Design review of the part built by this model. Coordinates are the model's own, in mm. A direction names the side the tool comes from. Round coordinates to 2 decimals unless told otherwise and drop trailing zeros. Order: outer loops, then holes, each group sorted by start corner. A loop starts at its lowest first (then second) coordinate and runs counter-clockwise, first axis right, second up. Notation, with made-up numbers: M -23.75,89.5 L 18.25,89.5 A8 cw 18.25,102.5 Z; hole C -9,-38.75 d7. An arc over 180 degrees is marked long. Use a Markdown table: item, result. Add a question column.
(1) Take a section at B-B (y = 0). Write out the cut boundary in (x, z).
(2) The part is to be moulded in two halves that separate along Z. For faces 4 (the face through (2.521, -48.656, 1.084)), 5 (the face through (-4, -36, 0)), 6 (the face through (0.06, -15.57, 7.88)), say which applies: released by +Z, released by -Z, zero draft, split by the parting line, or undercut.
(3) Take a section at C-C (x = -2). Write out the cut boundary in (y, z).
(4) Take a section at A-A (z = 0). Write out the cut boundary in (x, y).
(5) Take a section at D-D (y = -40). Write out the cut boundary in (x, z).
(6) To check wall thickness, follow probe 1 along Y at (x, z) = (1.8, 0); probe 2 along X at (y, z) = (-38, -7); probe 3 along Y at (x, z) = (0, -12.5). State the ranges of each line that lie inside material, in increasing order. Write a range as from..to.
(7) Machinability: for faces 1 (the face through (1, -42.6, 1.2)), 2 (the face through (0, -22, 7)), 3 (the face through (0.06, -15.57, -7.88)), which of the approach directions +Z, -Z, +X, -X, +Y, -Y give a long, thin tool a straight path to every point of the face, cutting with its end or side? Answer none if there is none.
(8) For pin 1 (2.5 mm diameter, centred on y = -43.77, z = 0, fed in from +X); pin 2 (2.5 mm diameter, centred on x = -0.5, y = -73.5, fed in from -Z); pin 3 (3.5 mm diameter, centred on x = 0, y = -22, fed in from +Z); pin 4 (8 mm diameter, centred on y = -43.77, z = 0, fed in from +X), all flat-tipped, find the tip position at first contact; note any pin that passes through.
```python
from build123d import *

# Parameters (mm, degrees)
BOSS_EXTRUDE1_DEPTH      = 4
BOSS_EXTRUDE1_DEPTH_BACK = 4
FILLET1_R                = 10
SKETCH2_R                = 5
CUT_EXTRUDE1_DEPTH       = 3
SKETCH3_R                = 1.5
CUT_EXTRUDE2_DEPTH       = 5
SKETCH4_R                = 18.5
CUT_EXTRUDE3_DEPTH       = 8
SKETCH5_R                = 21.5
SKETCH5_R_2              = 18.5
BOSS_EXTRUDE2_DEPTH      = 7


with BuildPart() as part:
    # Sketch1 → Boss-Extrude1 (new, two sides: drawn at the far end of the back side and taken through both)
    with BuildSketch(Plane(origin=(0, 0, 0), x_dir=(0, 0, -1), z_dir=(1, 0, 0)).offset(-BOSS_EXTRUDE1_DEPTH_BACK)):
        with BuildLine():
            Line((-7, -14.38749457), (-7, -29.38749457))
            ThreePointArc((-7, -29.38749457), (-16, -43.77498914), (-7, -58.16248371))
            Line((-7, -58.16248371), (-7, -88.16248371))
            ThreePointArc((-7, -88.16248371), (0, -129.99103506), (7, -88.16248371))
            Line((7, -88.16248371), (7, -58.16248371))
            ThreePointArc((7, -58.16248371), (16, -43.77498914), (7, -29.38749457))
            Line((7, -29.38749457), (7, -14.38749457))
            ThreePointArc((7, -14.38749457), (0, 16), (-7, -14.38749457))
        make_face()
    extrude(amount=BOSS_EXTRUDE1_DEPTH + BOSS_EXTRUDE1_DEPTH_BACK)

    # Fillet1
    fillet1_edges = [part.edges().sort_by_distance(p)[0] for p in [
        (0, -29.38749457, 7),
        (0, -14.38749457, 7),
        (0, -14.38749457, -7),
        (0, -29.38749457, -7),
        (0, -58.16248371, -7),
        (0, -88.16248371, -7),
        (0, -88.16248371, 7),
        (0, -58.16248371, 7),
    ]]
    fillet(fillet1_edges, radius=FILLET1_R)

    # Sketch2 → Cut-Extrude1 (cut)
    with BuildSketch(Plane(origin=(4, 0, 0), x_dir=(0, 0, -1), z_dir=(1, 0, 0))):
        Circle(SKETCH2_R)
        with Locations((0, -43.77498914)):
            Circle(SKETCH2_R)
    extrude(amount=-CUT_EXTRUDE1_DEPTH, mode=Mode.SUBTRACT)

    # Sketch3 → Cut-Extrude2 (cut)
    with BuildSketch(Plane(origin=(1, 0, 0), x_dir=(0, 0, -1), z_dir=(1, 0, 0))):
        Circle(SKETCH3_R)
        with Locations((0, -43.77498914)):
            Circle(SKETCH3_R)
    extrude(amount=-CUT_EXTRUDE2_DEPTH, mode=Mode.SUBTRACT)

    # Sketch4 → Cut-Extrude3 (cut)
    with BuildSketch(Plane(origin=(4, 0, 0), x_dir=(0, 0, -1), z_dir=(1, 0, 0))):
        with Locations((0, -108.49103506)):
            Circle(SKETCH4_R)
    extrude(amount=-CUT_EXTRUDE3_DEPTH, mode=Mode.SUBTRACT)

    # Sketch5 → Boss-Extrude2 (add)
    with BuildSketch(Plane.ZY.offset(4)):
        with Locations(Location((0, -108.49103506, 0), (0, 0, 122.662030563))):
            Circle(SKETCH5_R)
        with Locations(Location((0, -108.49103506, 0), (0, 0, 180))):
            Circle(SKETCH5_R_2, mode=Mode.SUBTRACT)
    extrude(amount=BOSS_EXTRUDE2_DEPTH)


solid = part.part
```
Verdict:
| question | item | result |
|---|---|---|
| 1 | outline | M -4,-16 L 4,-16 L 4,-5 L 1,-5 L 1,-1.5 L -4,-1.5 Z; M -4,1.5 L 1,1.5 L 1,5 L 4,5 L 4,16 L -4,16 Z |
| 2 | face 4 | undercut |
| 2 | face 5 | zero draft |
| 2 | face 6 | released by +Z |
| 3 | outline | M -90.39,-11.6 A10 cw -81.97,-7 L -63.45,-7 A10 cw -55.88,-10.46 A16 ccw -31.67,-10.46 A10 cw -24.1,-7 L -19.67,-7 A10 cw -12.11,-10.46 A16 ccw long -12.11,10.46 A10 cw -19.67,7 L -24.1,7 A10 cw -31.67,10.46 A16 ccw -55.88,10.46 A10 cw -63.45,7 L -81.97,7 A10 cw -90.39,11.6 A21.5 ccw long Z; hole C -108.49,0 d37; hole C -43.77,0 d3; hole C 0,0 d3 |
| 4 | outline | M -11,-129.99 L 4,-129.99 L 4,-126.99 L -11,-126.99 Z; M -11,-89.99 L 4,-89.99 L 4,-48.77 L 1,-48.77 L 1,-45.27 L -4,-45.27 L -4,-86.99 L -11,-86.99 Z; M -4,-42.27 L 1,-42.27 L 1,-38.77 L 4,-38.77 L 4,-5 L 1,-5 L 1,-1.5 L -4,-1.5 Z; M -4,1.5 L 1,1.5 L 1,5 L 4,5 L 4,16 L -4,16 Z |
| 5 | outline | M -4,-15.55 L 4,-15.55 L 4,-3.28 L 1,-3.28 L 1,3.28 L 4,3.28 L 4,15.55 L -4,15.55 Z |
| 6 | probe 1 | y = -129.99..-126.99, -89.99..-48.77, -38.77..-5, 5..16 |
| 6 | probe 2 | x = -4..4 |
| 6 | probe 3 | y = -125.98..-122.13, -94.85..-91, -53.76..-33.79, -9.99..9.99 |
| 7 | face 1 | +X |
| 7 | face 2 | +Z, +X, -X |
| 7 | face 3 | -Z, +X, -X |
| 8 | pin 1 | passes through |
| 8 | pin 2 | stops at z = -7 |
| 8 | pin 3 | stops at z = 7 |
| 8 | pin 4 | stops at x = 1 |
